The drawing under review shows one solid part. Ordinate dimensions are in mm from its lowest x, y, z. Round coordinates to 2 decimals unless told otherwise and drop trailing zeros. Order: outer loops, then holes, each group sorted by start corner. A loop starts at its lowest first (then second) coordinate and runs counter-clockwise, first axis right, second up. Notation, with made-up numbers: M 58,-8 L 70,-8 A20 ccw 70,-3 Z; hole C 25,88.25 d4. An arc over 180 degrees is marked long. Answer as a JSON object with one key per item and string values. Group by question number.
1. Add section C-C on y = 7.5. State the section outline as (x, z) points, and give its area (3 significant figures).
2. To check wall thickness, follow probe 1 along Y at (x, z) = (18, 29); probe 2 along Y at (x, z) = (59, 16); probe 3 along X at (y, z) = (8.75, 31). State the ranges of each line that lie inside material, in increasing order. Write a range as [from, to].
3. Add section A-A on x = 28. State the section outline as (y, z) points.
4. Add section B-B on z = 25.4. State the section outline as (x, y) points.
5. Add section D-D on x = 49.5. State the section outline as (y, z) points, and give its area (3 significant figures).
6. Clearance check with a flat-ended pin moving along its axis: P1, Ø4.5, axis at x = 51, z = 10, coming from the +Y side. State where the tip first meets the part, or that it passes through.
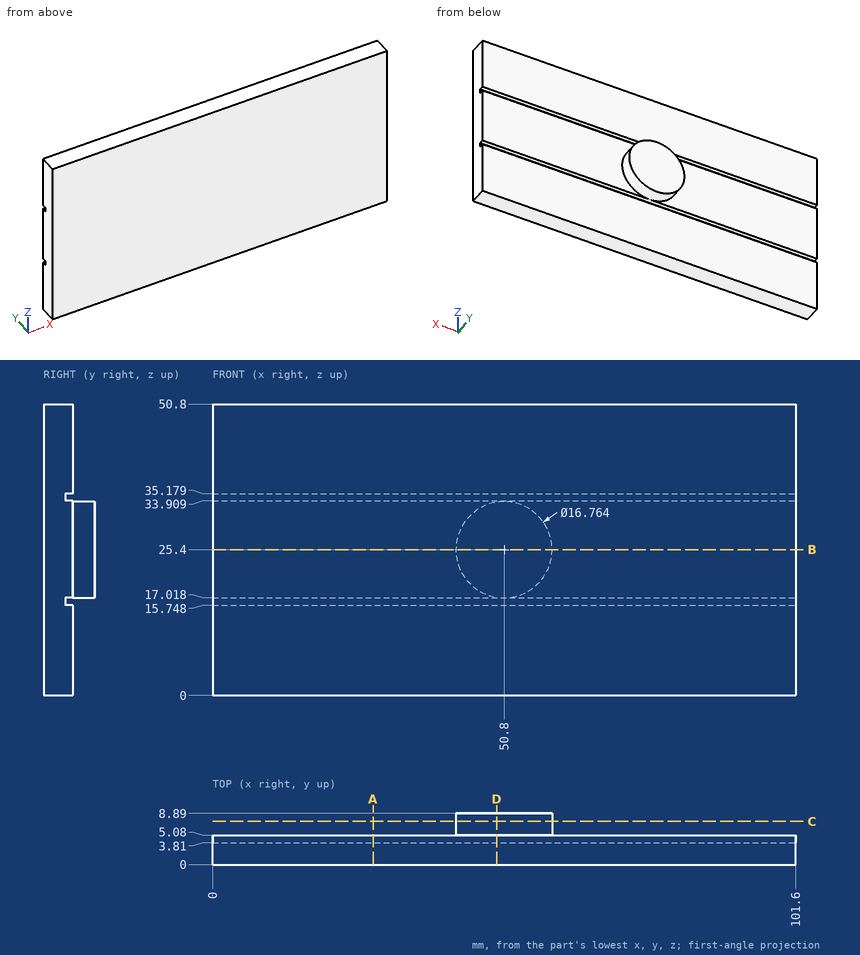
Recorded:
{
 "1": {"outline": "C 50.8,25.4 d16.76", "area": "221 mm²"},
 "2": {"probe 1": "y = [0, 5.08]", "probe 2": "y = [0, 3.81]", "probe 3": "x = [44.56, 57.04]"},
 "3": {"outline": "M 0,0 L 5.08,0 L 5.08,15.75 L 3.81,15.75 L 3.81,17.02 L 5.08,17.02 L 5.08,33.91 L 3.81,33.91 L 3.81,35.18 L 5.08,35.18 L 5.08,50.8 L 0,50.8 Z"},
 "4": {"outline": "M 0,0 L 101.6,0 L 101.6,5.08 L 59.18,5.08 L 59.18,8.89 L 42.42,8.89 L 42.42,5.08 L 0,5.08 Z"},
 "5": {"outline": "M 0,0 L 5.08,0 L 5.08,15.75 L 3.81,15.75 L 3.81,17.02 L 5.08,17.02 L 5.08,17.12 L 8.89,17.12 L 8.89,33.68 L 5.08,33.68 L 5.08,33.91 L 3.81,33.91 L 3.81,35.18 L 5.08,35.18 L 5.08,50.8 L 0,50.8 Z", "area": "318 mm²"},
 "6": {"P1": "stops at y = 5.08"}
}
